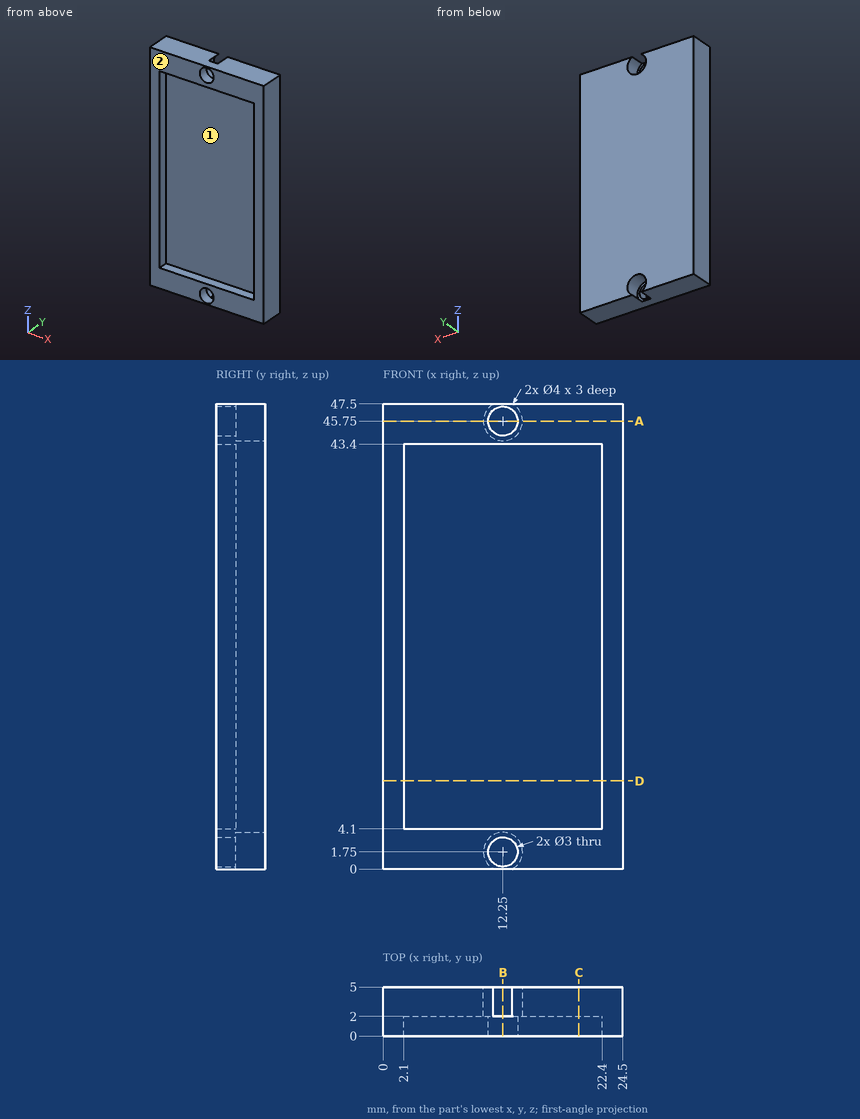
The figure shows three views and two pictorial views of one solid part (mm, origin at its lowest corner). Answer the questions. Round coordinates to 2 decimals unless told otherwise and drop trailing zeros. Write each loop counter-clockwise with the first axis right and the second up, starting at its lowest first coordinate (ties: lowest second). Pieces come first, ordered by that corner, then holes. Notation, with made-up numbers: (86.25, 63) -> (132.25, 63) arc R20 cw to (132.25, 91) -> close; hole circle Ø4 at (85, 75). An arc over 180 degrees is marked (long way). Answer as a JSON object with one key per item and string values. Group by question number.
Q1. Section D-D (z = 9) is taken. Write down the section's boundary in (x, y), plus the area to 3 significant figures.
Q2. Straight lines are drawn through the part: line 1 along Z through (x, y) = (12.25, 0.6); line 2 along X through (y, z) = (1.5, 21); line 3 along Z through (x, y) = (13.5, 3.4). For each, find the intervals that lie inside material, in ascending order.
Q3. Section A-A (z = 45.75) is taken. Write down the section's boundary in (x, y).
Q4. Section C-C (x = 20) is taken. Write down the section's boundary in (y, z), plus the area to 3 significant figures.
Q5. Determine the mould class of the marked faces 1 and 2 for opening direction Z: pulls with the +Z half, pulls with the -Z half, needs draft (parallel to the pull), parting line crosses it, or undercut.
Q6. Each of these flat-tipped pins is pushed along its axis until it touches: pin 1 Ø2.5 at (x, z) = (12.25, 1.75) entering from -Y; pin 2 Ø6 at (x, z) = (14, 22) entering from -Y; pin 3 Ø1.1 at (x, z) = (11.5, 2.5) entering from +Y. Where does it stop, or does it pass through?
Q7. Section B-B (x = 12.25) is taken. Write down the section's boundary in (y, z).
Check values:
{
 "1": {"outline": "(0, 0) -> (2.1, 0) -> (2.1, 2) -> (22.4, 2) -> (22.4, 0) -> (24.5, 0) -> (24.5, 5) -> (0, 5) -> close", "area": "81.9 mm^2"},
 "2": {"line 1": "0 to 0.25, 3.25 to 4.1, 43.4 to 44.25, 47.25 to 47.5", "line 2": "0 to 2.1, 22.4 to 24.5", "line 3": "0 to 0.19, 3.31 to 44.19, 47.31 to 47.5"},
 "3": {"outline": "(0, 0) -> (10.75, 0) -> (10.75, 2) -> (10.25, 2) -> (10.25, 5) -> (0, 5) -> close; (13.75, 0) -> (24.5, 0) -> (24.5, 5) -> (14.25, 5) -> (14.25, 2) -> (13.75, 2) -> close"},
 "4": {"outline": "(0, 0) -> (5, 0) -> (5, 47.5) -> (0, 47.5) -> (0, 43.4) -> (2, 43.4) -> (2, 4.1) -> (0, 4.1) -> close", "area": "159 mm^2"},
 "5": {"face 1": "undercut", "face 2": "needs draft"},
 "6": {"pin 1": "through", "pin 2": "y = 2", "pin 3": "y = 2"},
 "7": {"outline": "(0, 0) -> (2, 0) -> (2, 0.25) -> (0, 0.25) -> close; (0, 3.25) -> (2, 3.25) -> (2, 3.75) -> (5, 3.75) -> (5, 43.75) -> (2, 43.75) -> (2, 44.25) -> (0, 44.25) -> (0, 43.4) -> (2, 43.4) -> (2, 4.1) -> (0, 4.1) -> close; (0, 47.25) -> (2, 47.25) -> (2, 47.5) -> (0, 47.5) -> close"}
}
